Input: part model. Units: mm. Frame: model coordinates. A direction names the side the tool comes from. Coordinates: 2 decimals unless noted, no trailing zeros. Write each loop counter-clockwise with the first axis right and the second up, starting at its lowest first coordinate (ties: lowest second). Pieces come first, ordered by that corner, then holes. Notation, with made-up numbers: (-24, -14) - (29, -14) arc R28 cw to (29, 25) - close; hole circle Ø9 at (70.5, 71.25). An arc over 180 degrees is marked (long way). Use a Markdown table: item, result. Add a question column.
Q1. Material intervals for probe 1 along Z at (x, y) = (0, 24.85); probe 2 along Y at (x, z) = (-9, -18); probe 3 along X at (y, z) = (-24, 0), sorted ascending. Write a range as from..to.
Q2. Set-up query: faces 1 (the face through (-3, 23.812, -1)), 2 (the face through (-11.92, 18.94, -47.71)). Return all of +Z, -Z, +X, -X, +Y, -Y with unobstructed straight access to the full face (end or side cutting, diameter ignored); none if empty.
Q3. Section query A-A (z = 0). Return the cut outline in (x, y).
Q4. Section query C-C (x = -6.75). Return the cut outline in (y, z), then the cut area to 3 significant figures.
Q5. Section query B-B (y = 0). Return the cut outline in (x, z).
Q6. Pin query (flat end, axial travel): P1, Ø4, axis at y = -19.05, z = 50.26, coming from the +X side. Return the tip coordinate at first contact, or that it passes through.
Q7. Section query D-D (x = 0). Give the number of separate pieces and of enclosed holes in the cut face, then the cut area to 3 significant figures.
Q8. Mould query, pull axis Y, two halves, no side actions, for faces 3 (the face through (-11.3, 2, 76.2)), 4 (the face through (11.9, 18.94, -47.71)), 5 (the face through (3, -25.4, -1)). Classes: released by +Y, released by -Y, zero draft, split by the parting line, or undercut.
Autodesk Inventor part; units mm, degrees
ref_plane "YZ Plane" through (0, 0, 0) normal (1, 0, 0) x (0, 1, 0)
ref_plane "XZ Plane" through (0, 0, 0) normal (0, 1, 0) x (-1, 0, 0)
ref_plane "XY Plane" through (0, 0, 0) normal (0, 0, 1) x (1, 0, 0)
sketch "Sketch1" plane through (0, 0, 0) normal (0, 0, 1) x (1, 0, 0)
  line L0 (-12.7, -25.4) -> (12.7, -25.4)
  line L1 (12.7, -25.4) -> (12.7, 25.4)
  line L2 (12.7, 25.4) -> (-12.7, 25.4)
  line L3 (-12.7, 25.4) -> (-12.7, -25.4)
  line L4 (-12.7, -25.4) -> (12.7, 25.4) construction
  line L5 (12.7, -25.4) -> (-12.7, 25.4) construction
  line L6 (-11.1125, 23.8125) -> (11.1125, 23.8125)
  line L7 (11.1125, 23.8125) -> (11.1125, -23.8125)
  line L8 (11.1125, -23.8125) -> (-11.1125, -23.8125)
  line L9 (-11.1125, -23.8125) -> (-11.1125, 23.8125)
  point P0 (0, 0)
  dimension "width" = 25.4
  dimension "height" = 50.8
  dimension "thickness" = 1.5875
extrude "Extrusion1" add sketch "Sketch1" along normal mid plane 152.4
sketch "Sketch2" plane through (-12.7, 25.4, 76.2) normal (0, 1, 0) x (1, 0, 0)
  line L0 (0, 152.4) -> (0, 0) construction
  line L1 (25.4, 0) -> (0, 0) construction
  line L2 (25.4, 152.4) -> (25.4, 0) construction
  line L3 (0, 152.4) -> (25.4, 152.4) construction
  line L4 (12.7, 136.525) -> (12.7, 15.875) construction
  point P0 (12.7, 76.2)
  point P1 (12.7, 76.2)
  point P2 (12.7, 76.2)
  dimension "d5" = 120.65
hole "Hole1" at (0, 25.4, -60.325) at (0, 25.4, 60.325) at (0, 25.4, 0) direction (0, -1, 0) diameter 5.1054 end through all
sketch "Sketch4" plane through (12.7, -25.4, 76.2) normal (1, 0, 0) x (0, 0, -1)
  circle A0 centre (76.2, 25.4) radius 53.75 construction
  line L0 (25.9391, 6.35) -> (126.4609, 6.35) construction
  line L1 (126.4609, 6.35) -> (126.4609, 44.45) construction
  line L2 (126.4609, 44.45) -> (25.9391, 44.45) construction
  line L3 (25.9391, 44.45) -> (25.9391, 6.35) construction
  line L4 (25.9391, 6.35) -> (126.4609, 44.45) construction
  line L5 (126.4609, 6.35) -> (25.9391, 44.45) construction
  line L6 (0, 0) -> (0, 50.8) construction
  dimension "d25" = 107.5
  dimension "d28" = 38.1
hole "Hole3" at (12.7, 19.05, 50.2609) at (12.7, 19.05, -50.2609) at (12.7, -19.05, -50.2609) at (12.7, -19.05, 50.2609) direction (-1, 0, 0) diameter 5.1054 end through all
sketch "Sketch5" plane through (12.7, -25.4, 76.2) normal (1, 0, 0) x (0, 0, -1)
  circle A0 centre (76.2, 25.4) radius 19.05
  dimension "d36" = 38.1
extrude "Extrusion2" cut sketch "Sketch5" against normal blind 25.4
sketch "Sketch3" plane through (12.7, -25.4, 76.2) normal (1, 0, 0) x (0, 0, -1)
  line L0 (25.9391, 44.45) -> (126.4609, 44.45) construction
  line L1 (126.4609, 44.45) -> (126.4609, 6.35) construction
  line L2 (126.4609, 6.35) -> (25.9391, 6.35) construction
  line L3 (25.9391, 6.35) -> (25.9391, 44.45) construction
  line L4 (25.9391, 44.45) -> (126.4609, 6.35) construction
  line L5 (126.4609, 44.45) -> (25.9391, 6.35) construction
  circle A0 centre (76.2, 25.4) radius 60 construction
  circle A1 centre (76.2, 25.4) radius 47.5 construction
  circle A2 centre (76.2, 25.4) radius 53.75 construction
  dimension "d16" = 107.5
  dimension "d14" = 120
  dimension "d15" = 95
  dimension "d17" = 38.1
properties part number "GP7-004" material "Aluminum 6061"
Values follow:
| question | item | result |
|---|---|---|
| 1 | probe 1 | -76.2..-62.88, -57.77..-2.55, 2.55..57.77, 62.88..76.2 |
| 1 | probe 2 | -25.4..-23.81, 23.81..25.4 |
| 1 | probe 3 | -12.7..-2.55, 2.55..12.7 |
| 2 | face 1 | +Z, -Z |
| 2 | face 2 | +X, -X |
| 3 | outline | (-12.7, -25.4) - (-2.55, -25.4) - (-2.55, -23.81) - (-11.11, -23.81) - (-11.11, -19.05) - (-12.7, -19.05) - close; (-12.7, 19.05) - (-11.11, 19.05) - (-11.11, 23.81) - (-2.55, 23.81) - (-2.55, 25.4) - (-12.7, 25.4) - close; (2.55, -25.4) - (12.7, -25.4) - (12.7, -19.05) - (11.11, -19.05) - (11.11, -23.81) - (2.55, -23.81) - close; (2.55, 23.81) - (11.11, 23.81) - (11.11, 19.05) - (12.7, 19.05) - (12.7, 25.4) - (2.55, 25.4) - close |
| 4 | outline | (-25.4, -76.2) - (-23.81, -76.2) - (-23.81, 76.2) - (-25.4, 76.2) - close; (23.81, -76.2) - (25.4, -76.2) - (25.4, 76.2) - (23.81, 76.2) - close |
| 4 | area | 484 mm2 |
| 5 | outline | (-12.7, -76.2) - (-11.11, -76.2) - (-11.11, -19.05) - (-12.7, -19.05) - close; (-12.7, 19.05) - (-11.11, 19.05) - (-11.11, 76.2) - (-12.7, 76.2) - close; (11.11, -76.2) - (12.7, -76.2) - (12.7, -19.05) - (11.11, -19.05) - close; (11.11, 19.05) - (12.7, 19.05) - (12.7, 76.2) - (11.11, 76.2) - close |
| 6 | P1 | through |
| 7 | separate pieces | 8 |
| 7 | enclosed holes | 0 |
| 7 | area | 435 mm2 |
| 8 | face 3 | zero draft |
| 8 | face 4 | undercut |
| 8 | face 5 | released by -Y |
